Autodesk Fusion 360 part; units mm, degrees
sketch "Sketch1" plane through (0, 0, 0) normal (0, 1, 0) x (1, 0, 0)
  line L0 (23.1297, 26.25) -> (-23.1297, 26.25)
  line L1 (-23.1297, 26.25) -> (-23.1297, -26.25)
  line L2 (-23.1297, -26.25) -> (23.1297, -26.25)
  line L3 (23.1297, -26.25) -> (23.1297, 26.25)
  line L4 (23.1297, 26.25) -> (-23.1297, -26.25) construction
  line L5 (-23.1297, 26.25) -> (23.1297, -26.25) construction
  line L6 (-20.1297, -18.25) -> (-7.1297, -18.25)
  line L7 (-7.1297, -18.25) -> (-7.1297, -13.25)
  line L8 (-7.1297, -13.25) -> (-20.1297, -13.25)
  line L9 (-20.1297, -13.25) -> (-20.1297, -18.25)
  circle A0 centre (-12.6297, 15.75) radius 7.5
  line L10 (-5.5297, -13.25) -> (-5.5297, -18.25)
  line L11 (7.4703, -13.25) -> (-5.5297, -13.25)
  line L12 (7.4703, -18.25) -> (7.4703, -13.25)
  line L13 (-5.5297, -18.25) -> (7.4703, -18.25)
  line L14 (-20.1297, -6.65) -> (-20.1297, -11.65)
  line L15 (-7.1297, -6.65) -> (-20.1297, -6.65)
  line L16 (-7.1297, -11.65) -> (-7.1297, -6.65)
  line L17 (-20.1297, -11.65) -> (-7.1297, -11.65)
  line L18 (-5.5297, -6.65) -> (-5.5297, -11.65)
  line L19 (7.4703, -6.65) -> (-5.5297, -6.65)
  line L20 (7.4703, -11.65) -> (7.4703, -6.65)
  line L21 (-5.5297, -11.65) -> (7.4703, -11.65)
  line L22 (-20.1297, -0.05) -> (-20.1297, -5.05)
  line L23 (-7.1297, -0.05) -> (-20.1297, -0.05)
  line L24 (-7.1297, -5.05) -> (-7.1297, -0.05)
  line L25 (-20.1297, -5.05) -> (-7.1297, -5.05)
  line L26 (-5.5297, -0.05) -> (-5.5297, -5.05)
  line L27 (7.4703, -0.05) -> (-5.5297, -0.05)
  line L28 (7.4703, -5.05) -> (7.4703, -0.05)
  line L29 (-5.5297, -5.05) -> (7.4703, -5.05)
  line L30 (-20.1297, 6.55) -> (-20.1297, 1.55)
  line L31 (-7.1297, 6.55) -> (-20.1297, 6.55)
  line L32 (-7.1297, 1.55) -> (-7.1297, 6.55)
  line L33 (-20.1297, 1.55) -> (-7.1297, 1.55)
  line L34 (-5.5297, 6.55) -> (-5.5297, 1.55)
  line L35 (7.4703, 6.55) -> (-5.5297, 6.55)
  line L36 (7.4703, 1.55) -> (7.4703, 6.55)
  line L37 (-5.5297, 1.55) -> (7.4703, 1.55)
  line L38 (7.4703, -18.25) -> (23.1297, -18.25) construction
  line L39 (17.2618, -18.25) -> (9.0703, -12.5142)
  line L40 (9.0703, -12.5142) -> (11.9382, -8.4185)
  line L41 (11.9382, -8.4185) -> (20.1297, -14.1542)
  line L42 (20.1297, -14.1542) -> (17.2618, -18.25)
  line L43 (17.2618, -10.514) -> (9.0703, -4.7782)
  line L44 (9.0703, -4.7782) -> (11.9382, -0.6825)
  line L45 (11.9382, -0.6825) -> (20.1297, -6.4182)
  line L46 (20.1297, -6.4182) -> (17.2618, -10.514)
  line L47 (17.2618, -2.778) -> (9.0703, 2.9578)
  line L48 (9.0703, 2.9578) -> (11.9382, 7.0535)
  line L49 (11.9382, 7.0535) -> (20.1297, 1.3178)
  line L50 (20.1297, 1.3178) -> (17.2618, -2.778)
  circle A1 centre (5.3703, 15.75) radius 7.5
  line L51 (20.1297, 23.25) -> (15.8797, 23.25)
  line L52 (15.8797, 23.25) -> (15.8797, 17.75)
  line L53 (15.8797, 17.75) -> (20.1297, 17.75)
  line L54 (20.1297, 17.75) -> (20.1297, 23.25)
  line L55 (20.1297, 23.25) -> (15.8797, 17.75) construction
  line L56 (15.8797, 23.25) -> (20.1297, 17.75) construction
  line L57 (20.1297, 10.65) -> (20.1297, 16.15)
  line L58 (15.8797, 16.15) -> (15.8797, 10.65)
  line L59 (15.8797, 10.65) -> (20.1297, 10.65)
  line L60 (20.1297, 16.15) -> (15.8797, 16.15)
  circle A2 centre (-18.6297, -23.25) radius 1.5
  line L61 (-23.1297, -20.25) -> (23.1297, -20.25)
  circle A3 centre (-6.2104, -23.25) radius 1.5
  circle A4 centre (6.209, -23.25) radius 1.5
  circle A5 centre (18.6283, -23.25) radius 1.5
  point P0 (18.0047, 20.5)
  dimension "d1" = 13
  dimension "d2" = 5
  dimension "d4" = 3
  dimension "d5" = 15
  dimension "d6" = 10.5
  dimension "d7" = 10.5
  dimension "d8" = 52.5
  dimension "d11" = 14.6
  dimension "d12" = 6.6
  dimension "d16" = 35
  dimension "d17" = 1.6
  dimension "d18" = 10
  dimension "d19" = 5
  dimension "d21" = 3
  dimension "d24" = 0
  dimension "d25" = 7.736
  dimension "d28" = 18
  dimension "d29" = 0
  dimension "d36" = 4.25
  dimension "d37" = 5.5
  dimension "d38" = 3
  dimension "d39" = 3
  dimension "d42" = 0
  dimension "d43" = -7.1
  dimension "d44" = 3
  dimension "d46" = 4.5
  dimension "d47" = 3
  dimension "d48" = 6
  dimension "d49" = 2
  dimension "d52" = 37.258
  dimension "d53" = 0
extrude "Extrude3" add sketch "Sketch1" along normal blind 3
extrude "Extrude4" add sketch "Sketch1" along normal blind 58 from surface at 3 contours L0 L1 L3 L61
extrude "Extrude5" add sketch "Sketch1" along normal blind 2 from surface at 61 contours L0 L1 L3 L61 | L6 L7 L8 L9 | A0 | L10 L11 L12 L13 | L14 L15 L16 L17 | L18 L19 L20 L21 | L22 L23 L24 L25 | L26 L27 L28 L29 | L30 L31 L32 L33 | L34 L35 L36 L37 | L39 L40 L41 L42 | L43 L44 L45 L46 | L47 L48 L49 L50 | A1 | L51 L52 L53 L54 | L57 L58 L59 L60
fillet "Fillet2" radius 5 6 edges at (23.1297, 1.5, 26.25) (23.1297, 33, 20.25) (-23.1297, 1.5, 26.25) (-23.1297, 33, 20.25) (23.1297, 31.5, -26.25) (-23.1297, 31.5, -26.25)
equation "d6 = 7.5 mm + 3 mm"
equation "d25 = 5.736 mm + 2 mm"
equation "d43 = -5.5 mm - 1.6 mm"
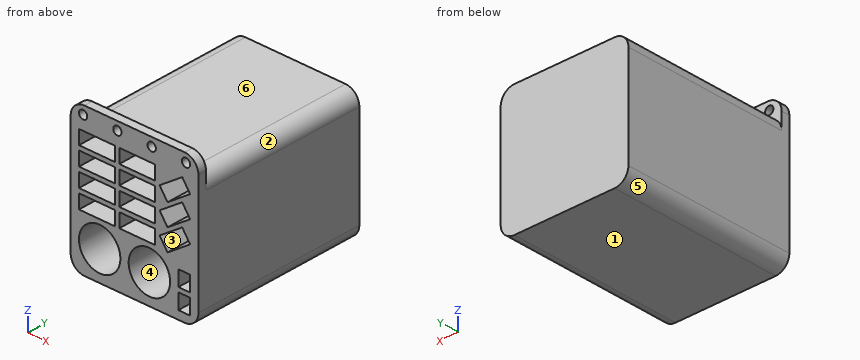
The model under review builds one solid part; all positions refer to its coordinate system, in mm. Face numbers are marked on the shaded views. A direction names the side the tool comes from. Round coordinates to 2 decimals unless told otherwise and drop trailing zeros. Write each loop counter-clockwise with the first axis right and the second up, starting at its lowest first coordinate (ties: lowest second). Pieces come first, ordered by that corner, then holes. Notation, with made-up numbers: (60, -8.75) - (74, -8.75) arc R20 cw to (74, 29.25) - close; hole circle Ø9 at (-14, 6.5). An arc over 180 degrees is marked (long way). Answer as CSV lines item,"result". Start each with the question number.
(1) To check wall thickness, follow line 1 (X direction, y = 45, z = -15.75); line 2 (Z direction, x = -3.5, y = 6.5); line 3 (Z direction, x = 5.5, y = 59). State the ranges of each line that lie inside material, in increasing order.
(2) Draft analysis for pull direction X (two halves, no side actions). For the marked faces 1, 2 and 3, state which applies: pulls with the +X half, pulls with the -X half, needs draft (parallel to the pull), parting line crosses it, or undercut.
(3) For pin 1 Ø1 at (x, y) = (12.5, 18) entering from +Z; pin 2 Ø1 at (x, z) = (17, 8) entering from -Y, all flat-tipped, find the tip position at first contact; note any pin that passes through.
(4) We need section A-A on z = 23.25. State the section outline as (x, y) points, plus the area to 3 significant figures.
(5) We need section C-C on z = 1.5. State the section outline as (x, y) points, plus the area to 3 significant figures.
(6) For the marked faces 4, 5 and 6, list the 3-axis set-ups (+Z, -Z, +X, -X, +Y, -Y) from which the entire face can be reached by the end or side of a thin tool; tool diameter is ignored.
(7) We need section D-D on x = 11. State the section outline as (y, z) points.
Worked answers:
1,line 1,"-23.13 to -20.13, -5.13 to -2.13, 12.87 to 15.88, 20.13 to 23.13"
1,line 2,"-26.25 to -6.55, -1.55 to 0.05, 5.05 to 6.65, 11.65 to 13.25, 18.25 to 20.25"
1,line 3,"-26.25 to -23.25, -8.25 to -6.55, -1.55 to 0.05, 5.05 to 6.65, 11.65 to 13.25, 18.25 to 20.25"
2,face 1,"needs draft"
2,face 2,"pulls with the +X half"
2,face 3,"undercut"
3,pin 1,"z = 20.25"
3,pin 2,"y = 61"
4,outline,"(-22.71, 0) - (-20.13, 0) - (-20.13, 3) - (-22.71, 3) - close; (-17.13, 0) - (-7.71, 0) - (-7.71, 3) - (-17.13, 3) - close; (-4.71, 0) - (4.71, 0) - (4.71, 3) - (-4.71, 3) - close; (7.71, 0) - (17.13, 0) - (17.13, 3) - (7.71, 3) - close; (20.13, 0) - (22.71, 0) - (22.71, 3) - (20.13, 3) - close"
4,area,"100 mm²"
5,outline,"(-23.13, 0) - (-20.13, 0) - (-20.13, 61) - (-7.13, 61) - (-7.13, 0) - (-5.53, 0) - (-5.53, 61) - (7.47, 61) - (7.47, 0) - (11.37, 0) - (11.37, 61) - (13.11, 61) - (13.11, 0) - (15.44, 0) - (15.44, 61) - (18.16, 61) - (18.16, 0) - (23.13, 0) - (23.13, 63) - (-23.13, 63) - close"
5,area,"1,060 mm²"
6,face 4,"-Y"
6,face 5,"-Z, -X, +Y, -Y"
6,face 6,"+Z, +X, -X, +Y"
7,outline,"(0, -26.25) - (63, -26.25) - (63, 20.25) - (3, 20.25) - (3, 26.25) - (0, 26.25) - (0, 13.87) - (61, 13.87) - (61, 9.76) - (0, 9.76) - (0, 6.13) - (61, 6.13) - (61, 2.02) - (0, 2.02) - (0, -1.61) - (61, -1.61) - (61, -5.71) - (0, -5.71) - (0, -10.79) - (61, -10.79) - (61, -20.71) - (0, -20.71) - close"
